Autodesk Inventor part; units mm, degrees
ref_plane "YZ Plane" through (0, 0, 0) normal (1, 0, 0) x (0, 1, 0)
ref_plane "XZ Plane" through (0, 0, 0) normal (0, 1, 0) x (-1, 0, 0)
ref_plane "XY Plane" through (0, 0, 0) normal (0, 0, 1) x (1, 0, 0)
sketch "Sketch1" plane through (0, 0, 0) normal (0, 0, 1) x (1, 0, 0)
  line L0 (0, 0) -> (44, 0)
  line L1 (44, 0) -> (44, 10)
  line L2 (44, 10) -> (0, 10)
  line L3 (0, 10) -> (0, 0)
  circle A0 centre (29.5, 5) radius 2.25
  circle A1 centre (14.5, 5) radius 2.25
  line L4 (14.5, 5) -> (29.5, 5) construction
  point P0 (0, 5)
  point P1 (22, 5)
  point P2 (22, 10)
  dimension "d0" = 10
  dimension "d1" = 44
  dimension "d2" = 4.5
  dimension "d13" = 4.5
  dimension "d14" = 15
extrude "Extrusion3" add sketch "Sketch1" along normal blind 6.5
sketch "Sketch3" plane through (0, 0, 6.5) normal (0, 0, 1) x (1, 0, 0)
  line L0 (0, 0) -> (44, 0)
  line L1 (44, 10) -> (0, 10)
  line L2 (6.5, 10) -> (14.5, 10)
  line L3 (14.5, 10) -> (14.5, 14.5)
  line L4 (12.5, 16.5) -> (8.5, 16.5)
  line L5 (6.5, 14.5) -> (6.5, 10)
  line L6 (29.5, 10) -> (37.5, 10)
  line L7 (37.5, 10) -> (37.5, 14.5)
  line L8 (35.5, 16.5) -> (31.5, 16.5)
  line L9 (29.5, 14.5) -> (29.5, 10)
  line L10 (6.5, 0) -> (14.5, 0)
  line L11 (14.5, 0) -> (14.5, -4.5)
  line L12 (12.5, -6.5) -> (8.5, -6.5)
  line L13 (6.5, -4.5) -> (6.5, 0)
  line L14 (29.5, 0) -> (37.5, 0)
  line L15 (37.5, 0) -> (37.5, -4.5)
  line L16 (35.5, -6.5) -> (31.5, -6.5)
  line L17 (29.5, -4.5) -> (29.5, 0)
  arc A0 (8.5, 16.5) -> (6.5, 14.5) centre (8.5, 14.5) ccw
  arc A1 (14.5, 14.5) -> (12.5, 16.5) centre (12.5, 14.5) ccw
  arc A2 (31.5, 16.5) -> (29.5, 14.5) centre (31.5, 14.5) ccw
  arc A3 (37.5, 14.5) -> (35.5, 16.5) centre (35.5, 14.5) ccw
  arc A4 (6.5, -4.5) -> (8.5, -6.5) centre (8.5, -4.5) ccw
  arc A5 (12.5, -6.5) -> (14.5, -4.5) centre (12.5, -4.5) ccw
  arc A6 (29.5, -4.5) -> (31.5, -6.5) centre (31.5, -4.5) ccw
  arc A7 (35.5, -6.5) -> (37.5, -4.5) centre (35.5, -4.5) ccw
  line L18 (14.5, 12.5251) -> (29.5, 12.5251) construction
  point P0 (22, 12.5251)
  point P1 (22, 10)
  dimension "d17" = 2
  dimension "d18" = 8
  dimension "d19" = 8
  dimension "d20" = 6.5
  dimension "d21" = 6.5
  dimension "d22" = 15
extrude "Extrusion4" add sketch "Sketch3" against normal blind 6.5
equation "\"d20\" = d21"
properties part number "y_carriage_belt_mount_bed_holder" material "Plywood, Finish"
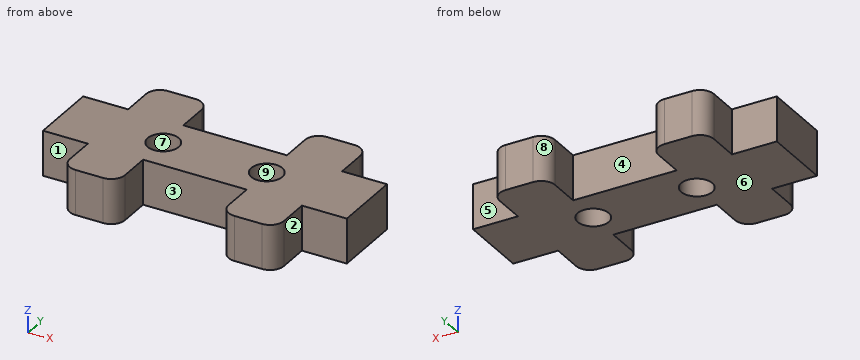
The listing builds one solid part. Answer for the finished solid, in the listing's coordinates (mm). Face numbers are marked on the shaded views. A direction names the side the tool comes from. Give positions to 0.01 mm unless a question says otherwise; leave off trailing zeros. Write each loop counter-clockwise with the first axis right and the second up, starting at its lowest first coordinate (ties: lowest second). Pieces come first, ordered by that corner, then holes. Notation, with made-up numbers: (4, 32.25) - (46, 32.25) arc R24 ccw to (46, 65.25) - close; hole circle Ø11 at (43, 26.25). An arc over 180 degrees is marked (long way). Use one line per item in the form item = value. Start each with the question number.
1) The mould has two halves that part along Y. Classify the marked faces 6, 7, 8 and 9: pulls with the +Y half, pulls with the -Y half, needs draft (parallel to the pull), parting line crosses it, or undercut.
2) Find section C-C on z = 4. Count the separate pieces of the cut face and the enclosed holes in it, plus the area to 3 significant figures.
3) Find section D-D on x = 16. Determine the outline of the cut face in (y, z), plus the area to 3 significant figures.
4) Find section A-A on y = -2. Determine the outline of the cut face in (x, z), plus the area to 3 significant figures.
5) A tool of negligible diameter and unlimited length cuts with its end or side. For the marked faces 1, 2, 3, 4 and 5, from which of +Z, -Z, +X, -X, +Y, -Y can it reach the whole face along a straight path? Write none if from no direction.
6) Flat-ended cylindrical pins translate along their axes: pin 1 Ø1.3 at (y, z) = (12, 2) entering from +X; pin 2 Ø2.5 at (x, y) = (29.5, 5) entering from +Z; pin 3 Ø3 at (x, z) = (40, 2.5) entering from -Y; pin 4 Ø2 at (x, z) = (40, 2.5) entering from +Y. Find the tip coordinate at first contact, or state that the pin passes through.
7) Consider line 1 along X through (y, z) = (6, 1.5); line 2 along X through (y, z) = (-4, 1); line 3 along X through (y, z) = (5.25, 3.25). Determine where each line is inside the solid, lowest interval first. Write a range as from..to.
8) Find section B-B on y = 5. Determine the outline of the cut face in (x, z), plus the area to 4 significant figures.
Geometry results:
q1.face_6 = needs draft
q1.face_7 = undercut
q1.face_8 = pulls with the +Y half
q1.face_9 = undercut
q2.separate_pieces = 1
q2.enclosed_holes = 2
q2.area = 609 mm2
q3.outline = (0, 0) - (3.32, 0) - (3.32, 6.5) - (0, 6.5) - close; (6.68, 0) - (10, 0) - (10, 6.5) - (6.68, 6.5) - close
q3.area = 43.2 mm2
q4.outline = (6.5, 0) - (14.5, 0) - (14.5, 6.5) - (6.5, 6.5) - close; (29.5, 0) - (37.5, 0) - (37.5, 6.5) - (29.5, 6.5) - close
q4.area = 104 mm2
q5.face_1 = +Z, -Z, -X, -Y
q5.face_2 = +Z, -Z, +X, -Y
q5.face_3 = +Z, -Z, -Y
q5.face_4 = +Z, -Z, +Y
q5.face_5 = +Z, -Z, +X, +Y
q6.pin_1 = 37.5
q6.pin_2 = through
q6.pin_3 = 0
q6.pin_4 = 10
q7.line_1 = 0..12.48, 16.52..27.48, 31.52..44
q7.line_2 = 6.5..14.5, 29.5..37.5
q7.line_3 = 0..12.26, 16.74..27.26, 31.74..44
q8.outline = (0, 0) - (12.25, 0) - (12.25, 6.5) - (0, 6.5) - close; (16.75, 0) - (27.25, 0) - (27.25, 6.5) - (16.75, 6.5) - close; (31.75, 0) - (44, 0) - (44, 6.5) - (31.75, 6.5) - close
q8.area = 227.5 mm2
